Geometry check sheet. Reference: the model listing, model coordinates, mm. A direction names the side the tool comes from. Coordinates: 2 decimals unless noted, no trailing zeros. Order: outer loops, then holes, each group sorted by start corner. A loop starts at its lowest first (then second) coordinate and runs counter-clockwise, first axis right, second up. Notation, with made-up numbers: (58, -19.75) - (69, -19.75) arc R16 cw to (69, -15.75) - close; hole circle Ø7 at (-15, -23). An arc over 180 degrees is marked (long way). Return JSON: item names as keys, results as strings. Group by question number.
Item 1: Draft check along Z on faces 5 (the cylindrical face through (8.506, 18.145, -36.96)), 6 (the flat face through (7, 11, -32.834)), 7 (the flat face through (3, 2.54, -12)), 8 (the cylindrical face through (4.671, 18.095, 8.745)). Enter one of: pulls with the +Z half, pulls with the -Z half, needs draft (parallel to the pull), parting line crosses it, or undercut.
Item 2: Gauge pin test, flat ends, axial feed: pin 1 (1 mm diameter, centred on x = -1.5, y = 12, fed in from -Z); pin 2 (2 mm diameter, centred on x = -1, y = 11, fed in from +Z); pin 3 (10 mm diameter, centred on y = 15, z = -9, fed in from +X). Record the tip position at first contact, or that the pin passes through.
Item 3: Section check C-C on x = -1. Enter the section's corners in (y, z) (3 decimals), then the cut area to 3 significant figures.
Item 4: Section check A-A on y = 6.75. Enter the section's corners in (x, z) (3 decimals), then the cut area to 3 significant figures.
Item 5: Scan lines: probe 1 along X at (y, z) = (13.5, -16); probe 2 along Y at (x, z) = (1, -32.5); probe 3 along Z at (x, y) = (4.5, 7.5). Record each from-to range of solid material in increasing order.
Item 6: Section check B-B on z = -12.5. Enter the section's corners in (x, y) (3 decimals).
Item 7: Section check D-D on z = 9. Enter the section's corners in (x, y) (3 decimals).
Item 8: Tool access check on faces 1 (the flat face through (-1, 9, -22.039)), 2 (the cylindrical face through (-4.169, 9.301, -21.134)), 3 (the flat face through (3.766, 9, 9)), 4 (the cylindrical face through (4.67, 9.3, 11.93)). Record the directions out of +Z, -Z, +X, -X, +Y, -Y that give a thin tool (end or side, any length) a straight path to the whole face; none if there is none.
Autodesk Inventor part; units mm, degrees
ref_plane "YZ Plane" through (0, 0, 0) normal (1, 0, 0) x (0, 1, 0)
ref_plane "XZ Plane" through (0, 0, 0) normal (0, 1, 0) x (-1, 0, 0)
ref_plane "XY Plane" through (0, 0, 0) normal (0, 0, 1) x (1, 0, 0)
sketch "Sketch1" plane through (0, 0, 0) normal (0, 1, 0) x (-1, 0, 0)
  line L0 (5.124, 12.8857) -> (-10.116, 12.8857)
  line L1 (-10.116, 12.8857) -> (-10.116, -37.9143)
  line L2 (-10.116, -37.9143) -> (5.124, -37.9143)
  line L3 (5.124, -37.9143) -> (5.124, 12.8857)
  line L4 (-10.116, 12.8857) -> (-3.766, 12.8857)
  line L5 (-3.766, 12.8857) -> (-3.766, 7.8057)
  line L6 (-3.766, 7.8057) -> (-10.116, 7.8057)
  line L7 (-10.116, 7.8057) -> (-10.116, 12.8857)
  line L8 (-10.116, -37.9143) -> (-3.766, -37.9143)
  line L9 (-3.766, -37.9143) -> (-3.766, -32.8343)
  line L10 (-3.766, -32.8343) -> (-10.116, -32.8343)
  line L11 (-10.116, -32.8343) -> (-10.116, -37.9143)
  line L12 (5.124, -2.9893) -> (0.044, -2.9893)
  line L13 (0.044, -2.9893) -> (0.044, -22.0393)
  line L14 (0.044, -22.0393) -> (5.124, -22.0393)
  line L15 (5.124, -22.0393) -> (5.124, -2.9893)
  point P0 (0, 0)
  dimension "d0" = 15.24
  dimension "d1" = 50.8
  dimension "d2" = 6.35
  dimension "d3" = 5.08
  dimension "d4" = 5.08
  dimension "d8" = 5.08
  dimension "d9" = 19.05
extrude "Extrusion1" add sketch "Sketch1" along normal blind 19.05 contours L5 L6 L1 L0 | L3 L14 L13 L12 | L10 L9 L2 L1
extrude "Extrusion2" add sketch "Sketch1" along normal blind 2.54 contours L3 L12 L13 L14 L2 L9 L10 L1 L6 L5 L0
fillet "Fillet1" radius 8.89 2 edges at (-5.124, 1.27, 12.8857) (-5.124, 1.27, -37.9143)
fillet "Fillet2" radius 3.175 11 edges at (-2.584, 19.05, -2.9893) (-5.124, 19.05, -12.5143) (-5.124, 10.795, -2.9893) (-5.124, 10.795, -22.0393) (-2.584, 19.05, -22.0393) (3.766, 10.795, 12.8857) (3.766, 19.05, 10.3457) (6.941, 19.05, 12.8857) (3.766, 19.05, -35.3743) (6.941, 19.05, -37.9143) (3.766, 10.795, -37.9143)
equation "\"BendRadius\" = Thickness"
equation "\"BendReliefWidth\" = Thickness"
equation "\"BendReliefDepth\" = 0.5 * Thickness"
equation "\"CornerReliefSize\" = 4 * Thickness"
equation "\"MinimumRemnant\" = 2 * Thickness"
equation "\"TransitionRadius\" = BendRadius"
equation "\"JacobiRadiusSize\" = BendRadius"
equation "\"GapSize\" = Thickness"
properties part number "BatteryStopper" material "ABS Plastic"
Computed:
{
 "1": {"face 5": "pulls with the -Z half", "face 6": "undercut", "face 7": "undercut", "face 8": "needs draft"},
 "2": {"pin 1": "stops at z = -22.04", "pin 2": "stops at z = -2.99", "pin 3": "stops at x = -0.04"},
 "3": {"outline": "(0, -36.529) - (2.54, -36.529) - (2.54, -22.039) - (15.875, -22.039) arc R3.175 ccw to (19.05, -18.864) - (19.05, -6.164) arc R3.175 ccw to (15.875, -2.989) - (2.54, -2.989) - (2.54, 11.5) - (0, 11.5) - close", "area": "432 mm²"},
 "4": {"outline": "(-5.124, -18.864) arc R3.175 ccw to (-1.949, -22.039) - (-0.044, -22.039) - (-0.044, -2.989) - (-1.949, -2.989) arc R3.175 ccw to (-5.124, -6.164) - close; (3.766, -34.739) arc R3.175 ccw to (6.941, -37.914) - (10.116, -37.914) - (10.116, -32.834) - (3.766, -32.834) - close; (3.766, 7.806) - (10.116, 7.806) - (10.116, 12.886) - (6.941, 12.886) arc R3.175 ccw to (3.766, 9.711) - close", "area": "153 mm²"},
 "5": {"probe 1": "x = -5.12 to -0.04", "probe 2": "y = 0 to 2.54", "probe 3": "z = -36.77 to -32.83, 7.81 to 11.74"},
 "6": {"outline": "(-5.124, 0) - (10.116, 0) - (10.116, 2.54) - (-0.044, 2.54) - (-0.044, 19.05) - (-1.949, 19.05) arc R3.175 ccw to (-5.124, 15.875) - close"},
 "7": {"outline": "(-3.582, 0) - (10.116, 0) - (10.116, 19.05) - (6.941, 19.05) arc R3.175 ccw to (3.766, 15.875) - (3.766, 2.54) - (-3.582, 2.54) - close"},
 "8": {"face 1": "-Z, +X, -X, +Y", "face 2": "-Z, -X, +Y", "face 3": "+Z, -Z, -X, +Y", "face 4": "+Z, -X, +Y"}
}
